from build123d import *

# Parameters (mm, degrees)
BOSS_EXTRUDE1_DEPTH = 15
SKETCH5_R           = 5
BOSS_EXTRUDE4_DEPTH = 22.5


with BuildPart() as part:
    # profiil → Boss-Extrude1 (new body)
    with BuildSketch(Plane.XY):
        with BuildLine():
            Line((35, 22.5), (17.5, 22.5))
            ThreePointArc((17.5, 22.5), (0, 5), (-17.5, 22.5))
            Line((-17.5, 22.5), (-35, 22.5))
            Line((-35, 22.5), (-35, 0))
            Line((-35, 0), (35, 0))
            Line((35, 0), (35, 22.5))
        make_face()
    extrude(amount=BOSS_EXTRUDE1_DEPTH)

    # Sketch5 → Boss-Extrude4 (add, through all)
    with BuildSketch(Plane(origin=(0, 0, 0), x_dir=(1, 0, 0), z_dir=(0, 1, 0))):
        with Locations((-25, -7.5)):
            Circle(SKETCH5_R)
        with Locations((25, -7.5)):
            Circle(SKETCH5_R)
    extrude(amount=BOSS_EXTRUDE4_DEPTH)


solid = part.part
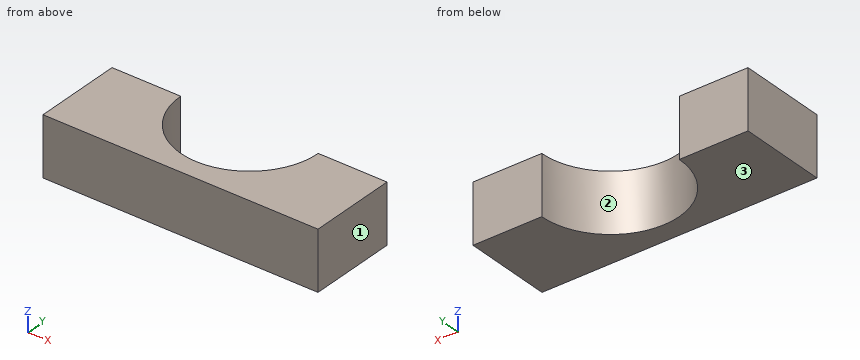
The listing builds one solid part. Answer for the finished solid, in the listing's coordinates (mm). Face numbers are marked on the shaded views. Coordinates: 2 decimals unless noted, no trailing zeros. Loops run counter-clockwise (first coordinate to the right, second up) from the corner with the lowest first, then second, coordinate; pieces in that order, holes last.
1) Find section B-B on z = 8. Write down the section's boundary in (x, y), then the cut area to 3 significant figures.
2) Find the intervals of material crossed by L1, parallel to X at y = 17.5, z = 4; L2, parallel to X at y = 14.5, z = 5; L3, parallel to Y at x = 2.5, z = 12.75, in increasing order.
3) Find section C-C on y = 17.5. Write down the section's boundary in (x, z).
4) Find section D-D on x = 12. Write down the section's boundary in (y, z).
5) Find section A-A on y = 12. Write down the section's boundary in (x, z), then the cut area to 3 significant figures.
6) Determine the mould class of the marked faces 1, 2 and 3 for opening direction X: pulls with the +X half, pulls with the -X half, needs draft (parallel to the pull), parting line crosses it, or undercut.
Values:
1. outline: (-35, 0) - (35, 0) - (35, 22.5) - (17.5, 22.5) arc R17.5 cw to (-17.5, 22.5) - (-35, 22.5) - close
1. area: 1,090 mm2
2. L1: x = -35 to -16.77, 16.77 to 35
2. L2: x = -35 to -15.56, 15.56 to 35
2. L3: y = 0 to 5.18
3. outline: (-35, 0) - (-16.77, 0) - (-16.77, 15) - (-35, 15) - close; (16.77, 0) - (35, 0) - (35, 15) - (16.77, 15) - close
4. outline: (0, 0) - (9.76, 0) - (9.76, 15) - (0, 15) - close
5. outline: (-35, 0) - (-14, 0) - (-14, 15) - (-35, 15) - close; (14, 0) - (35, 0) - (35, 15) - (14, 15) - close
5. area: 630 mm2
6. face 1: pulls with the +X half
6. face 2: undercut
6. face 3: needs draft
